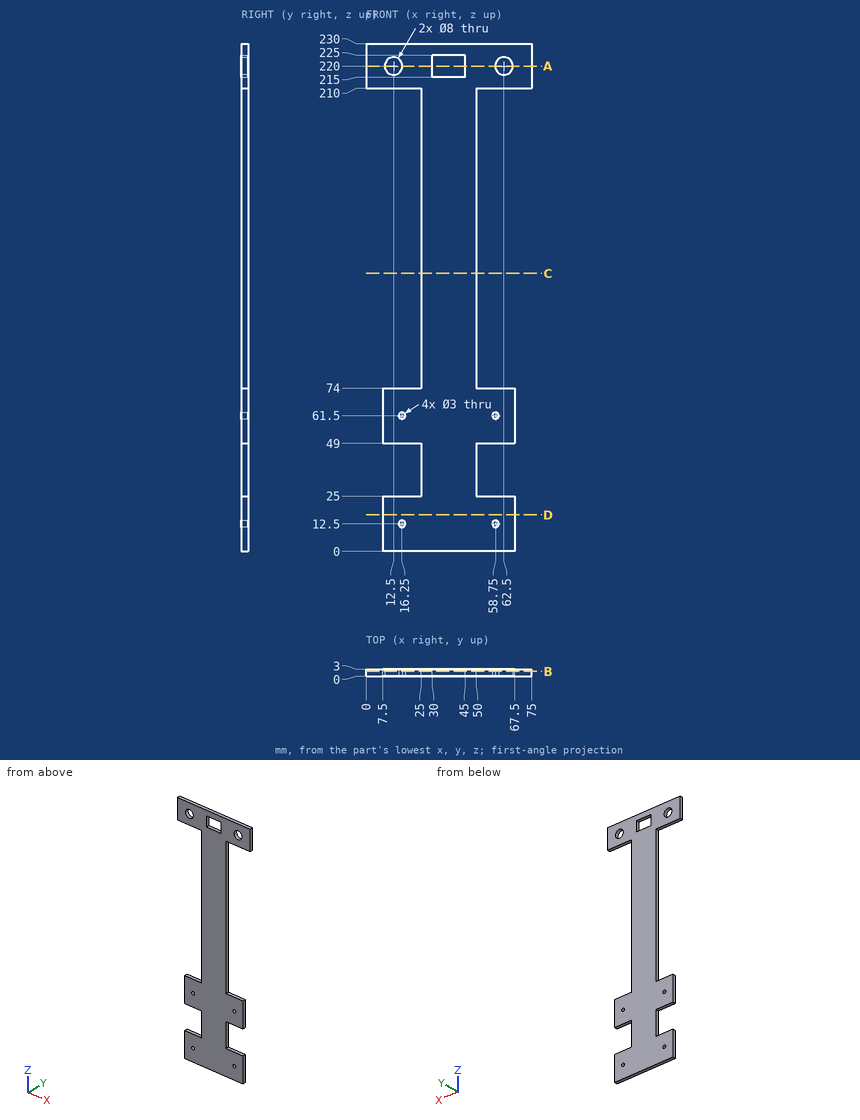
Verification items for this drawing (mm, ordinates from the low corner). Coordinates: 2 decimals unless noted, no trailing zeros. Loops run counter-clockwise (first coordinate to the right, second up) from the corner with the lowest first, then second, coordinate; pieces in that order, holes last.
Item 1: Sectioned sample at A-A, the plane z = 220. Record the boundary of the cut face in (x, y).
Item 2: Sectioned sample at C-C, the plane z = 126. Record the boundary of the cut face in (x, y).
Item 3: Sectioned sample at D-D, the plane z = 16.5. Record the boundary of the cut face in (x, y), then the cut area to 3 significant figures.
Item 4: Sectioned sample at B-B, the plane y = 2.1. Count the separate pieces of the cut face and the enclosed holes in it, then the cut area to 3 significant figures.
Item 5: Thickness scan on line 1 (Z direction, x = 62.5, y = 2.15); line 2 (X direction, y = 2.3, z = 12.5); line 3 (Z direction, x = 11, y = 0.6). Record the ranges inside material, lowest first.
Item 6: Go/stop test with flat-tipped pins: pin 1 Ø1.5 at (y, z) = (1, 59) entering from +X; pin 2 Ø0.9 at (y, z) = (1.5, 32) entering from -X; pin 3 Ø1 at (y, z) = (1.5, 195.5) entering from +X. Record where each tip stops, or that it passes through.
Check result:
1. outline: (0, 0) - (8.5, 0) - (8.5, 3) - (0, 3) - close; (16.5, 0) - (30, 0) - (30, 3) - (16.5, 3) - close; (45, 0) - (58.5, 0) - (58.5, 3) - (45, 3) - close; (66.5, 0) - (75, 0) - (75, 3) - (66.5, 3) - close
2. outline: (25, 0) - (50, 0) - (50, 3) - (25, 3) - close
3. outline: (7.5, 0) - (67.5, 0) - (67.5, 3) - (7.5, 3) - close
3. area: 180 mm2
4. separate pieces: 1
4. enclosed holes: 7
4. area: 8,220 mm2
5. line 1: z = 0 to 25, 49 to 74, 210 to 216, 224 to 230
5. line 2: x = 7.5 to 14.75, 17.75 to 57.25, 60.25 to 67.5
5. line 3: z = 0 to 25, 49 to 74, 210 to 216.29, 223.71 to 230
6. pin 1: stops at x = 67.5
6. pin 2: stops at x = 25
6. pin 3: stops at x = 50
